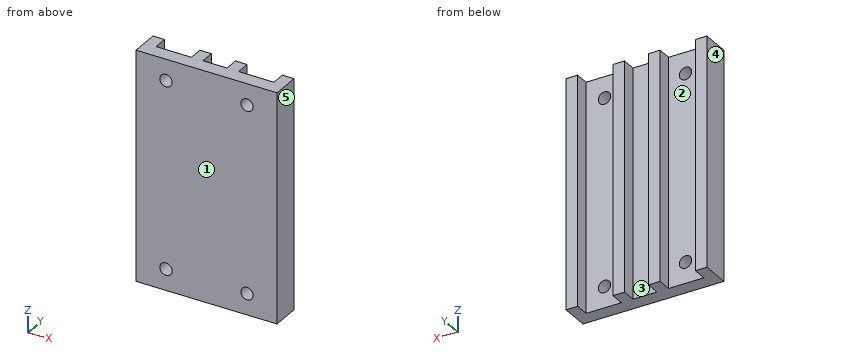
from build123d import *

# Parameters (mm, degrees)
SKETCH1_W           = 40
SKETCH1_H           = 65
SKETCH1_R           = 1.75
BOSS_EXTRUDE1_DEPTH = 4
SKETCH2_W           = 3.3
SKETCH2_H           = 65
BOSS_EXTRUDE2_DEPTH = 4


with BuildPart() as part:
    # Sketch1 → Boss-Extrude1 (new body)
    with BuildSketch(Plane(origin=(0, 0, 0), x_dir=(1, 0, 0), z_dir=(0, 1, 0))):
        Rectangle(SKETCH1_W, SKETCH1_H)
        with Locations((11.5, -26.5)):
            Circle(SKETCH1_R, mode=Mode.SUBTRACT)
        with Locations((-11.5, -26.5)):
            Circle(SKETCH1_R, mode=Mode.SUBTRACT)
        with Locations((11.5, 26.5)):
            Circle(SKETCH1_R, mode=Mode.SUBTRACT)
        with Locations((-11.5, 26.5)):
            Circle(SKETCH1_R, mode=Mode.SUBTRACT)
    extrude(amount=BOSS_EXTRUDE1_DEPTH)

    # Sketch2 → Boss-Extrude2 (add)
    with BuildSketch(Plane(origin=(0, 4, 0), x_dir=(1, 0, 0), z_dir=(0, 1, 0))):
        with Locations((-18.35, 0)):
            Rectangle(SKETCH2_W, SKETCH2_H)
        with Locations((18.35, 0)):
            Rectangle(SKETCH2_W, SKETCH2_H)
        with Locations((-5.05, 0)):
            Rectangle(SKETCH2_W, SKETCH2_H)
        with Locations((5.05, 0)):
            Rectangle(SKETCH2_W, SKETCH2_H)
    extrude(amount=BOSS_EXTRUDE2_DEPTH)


solid = part.part
Part model, mm, in its own coordinate system. Face numbers are marked on the shaded views. A direction names the side the tool comes from. Coordinates: 2 decimals unless noted, no trailing zeros. Order: outer loops, then holes, each group sorted by start corner. A loop starts at its lowest first (then second) coordinate and runs counter-clockwise, first axis right, second up. Notation, with made-up numbers: M 73,6 L 80,6 A10 ccw 80,18 Z; hole C 76,20 d3. An arc over 180 degrees is marked long. Use a Markdown table: item, result.
(1) Tool access for the marked faces 1 and 2: list every direction of +Z, -Z, +X, -X, +Y, -Y with a clear straight run to the whole face (end or side of a thin tool).
A:
| item | result |
|---|---|
| face 1 | +Z, -Z, +X, -X, -Y |
| face 2 | +Z, -Z, +Y |
(2) Cut at B-B on z = 26.5. Write the cut outline in (x, y), then the cut area to 3 significant figures.
A:
| item | result |
|---|---|
| outline | M -20,0 L -13.25,0 L -13.25,4 L -16.7,4 L -16.7,8 L -20,8 Z; M -9.75,0 L 9.75,0 L 9.75,4 L 6.7,4 L 6.7,8 L 3.4,8 L 3.4,4 L -3.4,4 L -3.4,8 L -6.7,8 L -6.7,4 L -9.75,4 Z; M 13.25,0 L 20,0 L 20,8 L 16.7,8 L 16.7,4 L 13.25,4 Z |
| area | 185 mm^2 |
(3) Cut at C-C on z = 15. Write the cut outline in (x, y), then the cut area to 3 significant figures.
A:
| item | result |
|---|---|
| outline | M -20,0 L 20,0 L 20,8 L 16.7,8 L 16.7,4 L 6.7,4 L 6.7,8 L 3.4,8 L 3.4,4 L -3.4,4 L -3.4,8 L -6.7,8 L -6.7,4 L -16.7,4 L -16.7,8 L -20,8 Z |
| area | 213 mm^2 |
(4) Flat gauge pins, fed straight in: pin 1 (2 mm diameter, centred on x = 11.5, z = -26.5, fed in from -Y); pin 2 (5 mm diameter, centred on x = -13, z = -1, fed in from +Y). Where does each tip first touch, or does it go through?
A:
| item | result |
|---|---|
| pin 1 | passes through |
| pin 2 | stops at y = 4 |
(5) Cut at A-A on x = -11.5. Write the cut outline in (y, z).
A:
| item | result |
|---|---|
| outline | M 0,-32.5 L 4,-32.5 L 4,-28.25 L 0,-28.25 Z; M 0,-24.75 L 4,-24.75 L 4,24.75 L 0,24.75 Z; M 0,28.25 L 4,28.25 L 4,32.5 L 0,32.5 Z |
(6) Pull direction X, two halves, no side cores. Call the marked faces 3, 4 and 5: released by +X, released by -X, zero draft, split by the parting line, or undercut.
A:
| item | result |
|---|---|
| face 3 | undercut |
| face 4 | released by -X |
| face 5 | released by +X |
(7) Probe L1, parallel to Z at x = -11.5, y = 3.2; L2, parallel to X at y = 2.4, z = -26.5; L3, parallel to X at y = 4.5, z = 4.5. List the from-to ranges inside material, lowest first.
A:
| item | result |
|---|---|
| L1 | z = -32.5 to -28.25, -24.75 to 24.75, 28.25 to 32.5 |
| L2 | x = -20 to -13.25, -9.75 to 9.75, 13.25 to 20 |
| L3 | x = -20 to -16.7, -6.7 to -3.4, 3.4 to 6.7, 16.7 to 20 |
